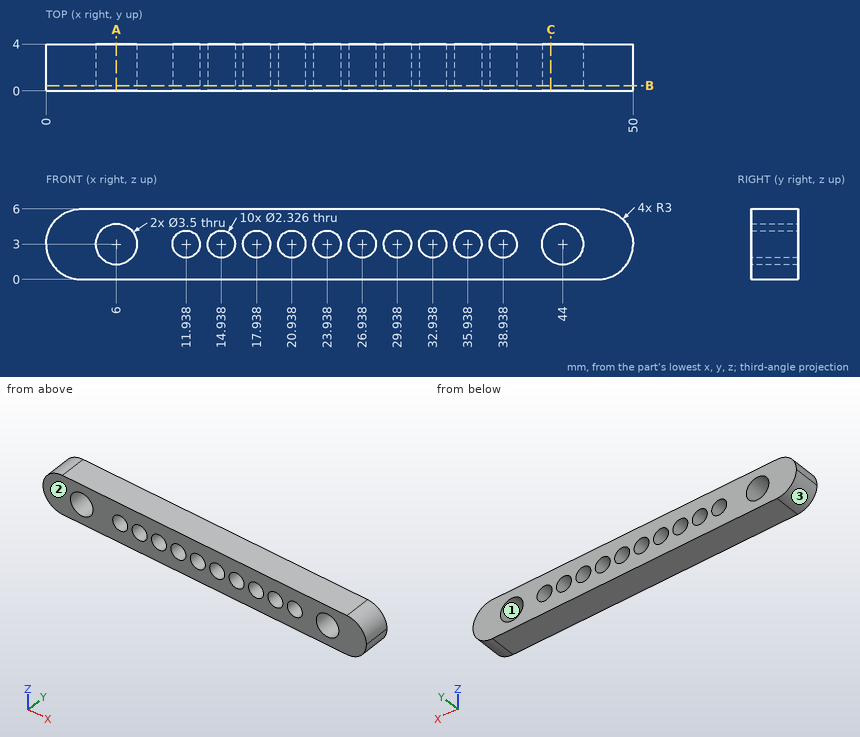
Verification items for this drawing (mm, ordinates from the low corner). Give positions to 0.01 mm unless a question says otherwise; leave off trailing zeros. Write each loop counter-clockwise with the first axis right and the second up, starting at its lowest first coordinate (ties: lowest second). Pieces come first, ordered by that corner, then holes.
1) Section check B-B, the plane y = 0.45. State how many separate pieces and enclosed holes the cut face has.
2) Section check C-C, the plane x = 43. Record the boundary of the cut face in (y, z).
3) Release check for a two-part mould opening along Z. For the marked faces 1, 2 and 3 record: pulls with the +Z half, pulls with the -Z half, needs draft (parallel to the pull), parting line crosses it, or undercut.
4) Gauge pin test, flat ends, axial feed: pin 1 (1.5 mm diameter, centred on y = 2, z = 0.5, fed in from +X); pin 2 (1 mm diameter, centred on x = 23.5, z = 2, fed in from -Y). Record the tip position at first contact, or that the pin passes through.
5) Material ranges on L1, parallel to X at y = 1.25, z = 1.5 (1 decimal); L2, parallel to Z at x = 36, y = 3.5; L3, parallel to Z at x = 39.5, y = 1.2, recorded low to high.
6) Section check A-A, the plane x = 6. Record the boundary of the cut face in (y, z).
Computed:
1. separate pieces: 1
1. enclosed holes: 12
2. outline: (0, 0) - (4, 0) - (4, 1.56) - (0, 1.56) - close; (0, 4.44) - (4, 4.44) - (4, 6) - (0, 6) - close
3. face 1: undercut
3. face 2: needs draft
3. face 3: pulls with the -Z half
4. pin 1: stops at x = 49.44
4. pin 2: stops at y = 0
5. L1: x = 0.4 to 5.1, 6.9 to 43.1, 44.9 to 49.6
5. L2: z = 0 to 1.84, 4.16 to 6
5. L3: z = 0 to 1.98, 4.02 to 6
6. outline: (0, 0) - (4, 0) - (4, 1.25) - (0, 1.25) - close; (0, 4.75) - (4, 4.75) - (4, 6) - (0, 6) - close
